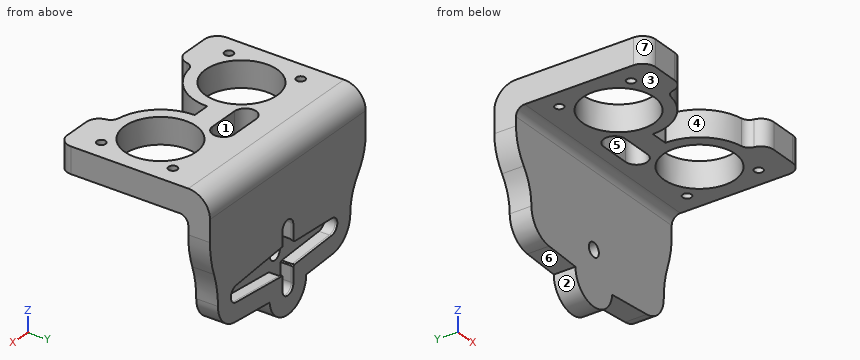
from build123d import *

# Parameters (mm, degrees)
EXTRUDE_THIN1_DEPTH = 5
BOSS_EXTRUDE1_DEPTH = 2
SKETCH3_R           = 1.6
CUT_EXTRUDE1_DEPTH  = 26.797771221
BOSS_EXTRUDE2_DEPTH = 5
SKETCH8_W           = 50
SKETCH8_H           = 6
BOSS_EXTRUDE6_DEPTH = 30
SKETCH10_R          = 8.25
SKETCH10_R_2        = 1
CUT_EXTRUDE2_DEPTH  = 55.037232534
FILLET2_R           = 5
FILLET4_R           = 3
EXTRUDE_THIN2_START = 4.5
EXTRUDE_THIN2_DEPTH = 0.5
FILLET5_R           = 2


# Read off the part's stored shape, not the designer's step: Extrude-Thin1, Boss-Extrude1, Extrude-Thin2
with BuildPart() as part:
    # Extrude-Thin1 outline → Extrude-Thin1 (new body)
    with BuildSketch(Plane(origin=(0, 0, 0), x_dir=(1, 0, 0), z_dir=(0, 1, 0))):
        with BuildLine():
            ThreePointArc((5.878005996, 6.958965141), (-0.252578975, 12.344591068), (-5.899998443, 6.454286146))
            Line((-5.899998443, 6.454286146), (-14.377365901, 5.991062641))
            ThreePointArc((-14.377365901, 5.991062641), (-20.05, 0), (-14.377365901, -5.991062641))
            Line((-14.377365901, -5.991062641), (-5.899998443, -6.454286146))
            ThreePointArc((-5.899998443, -6.454286146), (-0.252578975, -12.344591068), (5.878005996, -6.958965141))
            Line((5.878005996, -6.958965141), (16.97887538, -5.97664545))
            ThreePointArc((16.97887538, -5.97664545), (22.45, 0), (16.97887538, 5.97664545))
            Line((16.97887538, 5.97664545), (5.878005996, 6.958965141))
        make_face()
        with BuildLine():
            Line((-1.9, 2.87967012), (-1.9, 6.45))
            ThreePointArc((-1.9, 6.45), (0, 8.35), (1.9, 6.45))
            Line((1.9, 6.45), (1.9, 3.295349698))
            Line((1.9, 3.295349698), (16.626291793, 1.99221515))
            ThreePointArc((16.626291793, 1.99221515), (18.45, 0), (16.626291793, -1.99221515))
            Line((16.626291793, -1.99221515), (1.9, -3.295349698))
            Line((1.9, -3.295349698), (1.9, -6.45))
            ThreePointArc((1.9, -6.45), (0, -8.35), (-1.9, -6.45))
            Line((-1.9, -6.45), (-1.9, -2.87967012))
            ThreePointArc((-1.9, -2.87967012), (-2.057742861, -2.769150468), (-2.209072203, -2.65))
            Line((-2.209072203, -2.65), (-14.159121967, -1.99702088))
            ThreePointArc((-14.159121967, -1.99702088), (-16.05, 0), (-14.159121967, 1.99702088))
            Line((-14.159121967, 1.99702088), (-2.209072203, 2.65))
            ThreePointArc((-2.209072203, 2.65), (-2.057742861, 2.769150468), (-1.9, 2.87967012))
        make_face(mode=Mode.SUBTRACT)
    extrude(amount=EXTRUDE_THIN1_DEPTH)

    # Boss-Extrude1 outline → Boss-Extrude1 (add)
    with BuildSketch(Plane(origin=(0, 0, 0), x_dir=(1, 0, 0), z_dir=(0, 1, 0))):
        with BuildLine():
            ThreePointArc((1.9, 6.45), (0, 8.35), (-1.9, 6.45))
            Line((-1.9, 6.45), (-1.9, 2.87967012))
            ThreePointArc((-1.9, 2.87967012), (-2.057742861, 2.769150468), (-2.209072203, 2.65))
            Line((-2.209072203, 2.65), (-14.159121967, 1.99702088))
            ThreePointArc((-14.159121967, 1.99702088), (-16.05, 0), (-14.159121967, -1.99702088))
            Line((-14.159121967, -1.99702088), (-2.209072203, -2.65))
            ThreePointArc((-2.209072203, -2.65), (-2.057742861, -2.769150468), (-1.9, -2.87967012))
            Line((-1.9, -2.87967012), (-1.9, -6.45))
            ThreePointArc((-1.9, -6.45), (0, -8.35), (1.9, -6.45))
            Line((1.9, -6.45), (1.9, -3.295349698))
            Line((1.9, -3.295349698), (16.626291793, -1.99221515))
            ThreePointArc((16.626291793, -1.99221515), (18.45, 0), (16.626291793, 1.99221515))
            Line((16.626291793, 1.99221515), (1.9, 3.295349698))
            Line((1.9, 3.295349698), (1.9, 6.45))
        make_face()
    extrude(amount=BOSS_EXTRUDE1_DEPTH)

    # Sketch3 → Cut-Extrude1 (cut, through all)
    with BuildSketch(Plane(origin=(0, 2, 0), x_dir=(1, 0, 0), z_dir=(0, 1, 0))):
        with Locations(Location((0, 0, 0), (0, 0, 270))):
            Circle(SKETCH3_R)
    extrude(amount=-CUT_EXTRUDE1_DEPTH, mode=Mode.SUBTRACT)

    # Sketch4 → Boss-Extrude2 (add)
    # profile 1 of 2: a face of its own
    with BuildSketch(Plane.XZ):
        with BuildLine():
            Line((25, 25), (-25, 25))
            Line((-25, 25), (-25, 15))
            ThreePointArc((-25, 15), (-24.365263739, 11.051087966), (-22.525, 7.5))
            ThreePointArc((-22.525, 7.5), (-20.684736261, 3.948912034), (-20.05, 0))
            ThreePointArc((-20.05, 0), (-18.406844925, 4.125276027), (-14.377365901, 5.991062641))
            Line((-14.377365901, 5.991062641), (-5.899998443, 6.454286146))
            ThreePointArc((-5.899998443, 6.454286146), (-0.252578976, 12.344591068), (5.878005996, 6.958965141))
            Line((5.878005996, 6.958965141), (16.97887538, 5.97664545))
            ThreePointArc((16.97887538, 5.97664545), (20.875678043, 4.051342229), (22.45, 0))
            ThreePointArc((22.45, 0), (22.77102028, 3.803801552), (23.725, 7.5))
            ThreePointArc((23.725, 7.5), (24.67897972, 11.196198448), (25, 15))
            Line((25, 15), (25, 25))
        make_face()
    # profile 2 of 2: a face of its own
    with BuildSketch(Plane.XZ):
        with BuildLine():
            Line((-14.377365901, -5.991062641), (-5.899998443, -6.454286146))
            ThreePointArc((-5.899998443, -6.454286146), (-0.252578976, -12.344591068), (5.878005996, -6.958965141))
            Line((5.878005996, -6.958965141), (16.97887538, -5.97664545))
            ThreePointArc((16.97887538, -5.97664545), (22.45, 0), (16.97887538, 5.97664545))
            Line((16.97887538, 5.97664545), (5.878005996, 6.958965141))
            ThreePointArc((5.878005996, 6.958965141), (-0.252578976, 12.344591068), (-5.899998443, 6.454286146))
            Line((-5.899998443, 6.454286146), (-14.377365901, 5.991062641))
            ThreePointArc((-14.377365901, 5.991062641), (-20.05, 0), (-14.377365901, -5.991062641))
        make_face()
        with BuildLine():
            ThreePointArc((16.626291793, -1.99221515), (18.45, 0), (16.626291793, 1.99221515))
            Line((16.626291793, 1.99221515), (1.9, 3.295349698))
            Line((1.9, 3.295349698), (1.9, 6.45))
            ThreePointArc((1.9, 6.45), (0, 8.35), (-1.9, 6.45))
            Line((-1.9, 6.45), (-1.9, 2.87967012))
            ThreePointArc((-1.9, 2.87967012), (-2.057742862, 2.769150468), (-2.209072203, 2.65))
            Line((-2.209072203, 2.65), (-14.159121967, 1.99702088))
            ThreePointArc((-14.159121967, 1.99702088), (-16.05, 0), (-14.159121967, -1.99702088))
            Line((-14.159121967, -1.99702088), (-2.209072203, -2.65))
            ThreePointArc((-2.209072203, -2.65), (-2.057742862, -2.769150468), (-1.9, -2.87967012))
            Line((-1.9, -2.87967012), (-1.9, -6.45))
            ThreePointArc((-1.9, -6.45), (0, -8.35), (1.9, -6.45))
            Line((1.9, -6.45), (1.9, -3.295349698))
            Line((1.9, -3.295349698), (16.626291793, -1.99221515))
        make_face(mode=Mode.SUBTRACT)
    extrude(amount=-BOSS_EXTRUDE2_DEPTH)

    # Sketch8 → Boss-Extrude6 (add)
    with BuildSketch(Plane.XZ):
        with Locations((0, 22)):
            Rectangle(SKETCH8_W, SKETCH8_H)
    extrude(amount=BOSS_EXTRUDE6_DEPTH)

    # Sketch10 → Cut-Extrude2 (cut, through all)
    with BuildSketch(Plane.XY.offset(25)):
        with Locations((-13, -15)):
            Circle(SKETCH10_R)
        with Locations((13, -15)):
            Circle(SKETCH10_R)
        with Locations((20.5, -6.75)):
            Circle(SKETCH10_R_2)
        with Locations((20.5, -23.25)):
            Circle(SKETCH10_R_2)
        with Locations((-20.5, -23.25)):
            Circle(SKETCH10_R_2)
        with Locations((-20.5, -6.75)):
            Circle(SKETCH10_R_2)
        with BuildLine():
            Line((3.5, -9.8), (-3.5, -9.8))
            ThreePointArc((-3.5, -9.8), (-6, -7.3), (-3.5, -4.8))
            Line((-3.5, -4.8), (3.5, -4.8))
            ThreePointArc((3.5, -4.8), (6, -7.3), (3.5, -9.8))
        make_face()
        with BuildLine():
            Line((-2, -15), (2, -15))
            ThreePointArc((2, -15), (4.644900222, -22.154879991), (11.307692308, -25.869042951))
            ThreePointArc((11.307692308, -25.869042951), (12.519109051, -26.544345307), (13, -27.845232579))
            Line((13, -27.845232579), (13, -30))
            Line((13, -30), (-13, -30))
            Line((-13, -30), (-13, -27.845232579))
            ThreePointArc((-13, -27.845232579), (-12.519109051, -26.544345307), (-11.307692308, -25.869042951))
            ThreePointArc((-11.307692308, -25.869042951), (-4.644900222, -22.154879991), (-2, -15))
        make_face()
    extrude(amount=-CUT_EXTRUDE2_DEPTH, mode=Mode.SUBTRACT)

    # Fillet2
    fillet2_edges = [part.edges().sort_by_distance(p)[0] for p in [
        (0, 5, 25),
    ]]
    fillet(fillet2_edges, radius=FILLET2_R)

    # Fillet4
    fillet4_edges = [part.edges().sort_by_distance(p)[0] for p in [
        (25, -30, 22),
        (-25, -30, 22),
        (13, -30, 22),
        (-13, -30, 22),
    ]]
    fillet(fillet4_edges, radius=FILLET4_R)

    # Extrude-Thin2 outline → Extrude-Thin2 (add)
    with BuildSketch(Plane(origin=(0, 0, 0), x_dir=(1, 0, 0), z_dir=(0, 1, 0)).offset(EXTRUDE_THIN2_START)):
        with BuildLine():
            ThreePointArc((1.9, 6.45), (0, 8.35), (-1.9, 6.45))
            Line((-1.9, 6.45), (-1.9, 2.87967012))
            ThreePointArc((-1.9, 2.87967012), (-2.057742861, 2.769150468), (-2.209072203, 2.65))
            Line((-2.209072203, 2.65), (-14.159121967, 1.99702088))
            ThreePointArc((-14.159121967, 1.99702088), (-16.05, 0), (-14.159121967, -1.99702088))
            Line((-14.159121967, -1.99702088), (-2.209072203, -2.65))
            ThreePointArc((-2.209072203, -2.65), (-2.057742861, -2.769150468), (-1.9, -2.87967012))
            Line((-1.9, -2.87967012), (-1.9, -6.45))
            ThreePointArc((-1.9, -6.45), (0, -8.35), (1.9, -6.45))
            Line((1.9, -6.45), (1.9, -3.295349698))
            Line((1.9, -3.295349698), (16.626291793, -1.99221515))
            ThreePointArc((16.626291793, -1.99221515), (18.45, 0), (16.626291793, 1.99221515))
            Line((16.626291793, 1.99221515), (1.9, 3.295349698))
            Line((1.9, 3.295349698), (1.9, 6.45))
        make_face()
        with BuildLine():
            ThreePointArc((-1.75, -2.797766967), (-1.955868768, -2.657927268), (-2.150613493, -2.502970556))
            Line((-2.150613493, -2.502970556), (-14.15093782, -1.847244314))
            ThreePointArc((-14.15093782, -1.847244314), (-15.9, 0), (-14.15093782, 1.847244314))
            Line((-14.15093782, 1.847244314), (-2.150613493, 2.502970556))
            ThreePointArc((-2.150613493, 2.502970556), (-1.955868768, 2.657927268), (-1.75, 2.797766967))
            Line((-1.75, 2.797766967), (-1.75, 6.45))
            ThreePointArc((-1.75, 6.45), (0, 8.2), (1.75, 6.45))
            Line((1.75, 6.45), (1.75, 3.158037104))
            Line((1.75, 3.158037104), (16.613069909, 1.842799014))
            ThreePointArc((16.613069909, 1.842799014), (18.3, 0), (16.613069909, -1.842799014))
            Line((16.613069909, -1.842799014), (1.75, -3.158037104))
            Line((1.75, -3.158037104), (1.75, -6.45))
            ThreePointArc((1.75, -6.45), (0, -8.2), (-1.75, -6.45))
            Line((-1.75, -6.45), (-1.75, -2.797766967))
        make_face(mode=Mode.SUBTRACT)
    extrude(amount=EXTRUDE_THIN2_DEPTH)

    # Fillet5
    fillet5_edges = [part.edges().sort_by_distance(p)[0] for p in [
        (0, 0, 19),
    ]]
    fillet(fillet5_edges, radius=FILLET5_R)


solid = part.part
CAD build for the part. Positions are in the model's coordinates, mm. Face numbers are marked on the shaded views. A direction names the side the tool comes from. Round coordinates to 2 decimals unless told otherwise and drop trailing zeros. Write each loop counter-clockwise with the first axis right and the second up, starting at its lowest first coordinate (ties: lowest second). Pieces come first, ordered by that corner, then holes. Notation, with made-up numbers: M -19,-2.5 L -11,-2.5 A19 ccw -11,23.5 Z; hole C -17,83 d4. An arc over 180 degrees is marked long. Put each result on its own line as item: value. Start each with the question number.
1) Pin check, flat tips, straight feed: pin 1 Ø0.6 at (y, z) = (5, -4) entering from +X; pin 2 Ø0.6 at (y, z) = (5, 4.5) entering from +X; pin 3 Ø0.8 at (y, z) = (3, -5.5) entering from +X. Stop position of each tip, or through.
2) Saw through at A-A, the plane x = 0. Write the cut outline in (y, z).
3) Saw through at C-C, the plane x = 10. Write the cut outline in (y, z), and give its area (3 significant figures).
4) Saw through at B-B, the plane y = -21. Write the cut outline in (x, z).
5) 3-axis set-ups, long thin cutter, end or side, ignore diameter. For the marked faces 1, 2, 3 and 4: which of +Z, -Z, +X, -X, +Y, -Y reach the whole face in a straight line?
6) Pull direction Y, two halves, no side cores. Call the marked faces 5, 6 and 7: pulls with the +Y half, pulls with the -Y half, needs draft (parallel to the pull), parting line crosses it, or undercut.
7) Drill centre lines: probe 1 along X at (y, z) = (-6, 22); probe 2 along X at (y, z) = (-22.5, 20.5); probe 3 along Z at (x, y) = (-11, -25). Where is each one in solid material? Low to high. Write a range as [from, to].
8) Saw through at D-D, the plane z = -1. Write the cut outline in (x, y), and give its area (3 significant figures).
Resolved:
1. pin 1: x = 21.17
1. pin 2: x = 22.96
1. pin 3: x = 19.61
2. outline: M -15,19 L -9.8,19 L -9.8,25 L -15,25 Z; M -4.8,19 L -2,19 A2 cw 0,17 L 0,1.6 L 2,1.6 L 2,8.35 L 4.5,8.35 L 4.5,8.2 L 5,8.2 L 5,20 A5 ccw 0,25 L -4.8,25 Z; M 0,-12.35 L 5,-12.35 L 5,-8.2 L 4.5,-8.2 L 4.5,-8.35 L 2,-8.35 L 2,-1.6 L 0,-1.6 Z
3. outline: M -25.58,19 L -22.69,19 L -22.69,25 L -25.58,25 Z; M -7.31,19 L -2,19 A2 cw 0,17 L 0,-6.59 L 5,-6.59 L 5,-2.43 L 4.5,-2.43 L 4.5,-2.58 L 2,-2.58 L 2,2.58 L 4.5,2.58 L 4.5,2.43 L 5,2.43 L 5,20 A5 ccw 0,25 L -7.31,25 Z
3. area: 199 mm²
4. outline: M -25,19 L -18.66,19 L -18.66,25 L -25,25 Z; M -7.34,19 L -3.78,19 L -3.78,25 L -7.34,25 Z; M 3.78,19 L 7.34,19 L 7.34,25 L 3.78,25 Z; M 18.66,19 L 25,19 L 25,25 L 18.66,25 Z
5. face 1: +Z, -Z
5. face 2: -Z, +Y, -Y
5. face 3: -Z, +X, -X, -Y
5. face 4: +Z, -Z, -Y
6. face 5: undercut
6. face 6: needs draft
6. face 7: pulls with the -Y half
7. probe 1: [-25, -21.16], [-19.84, -5.64], [5.64, 19.84], [21.16, 25]
7. probe 2: [-25, -21.16], [-19.84, -16.44], [-9.56, -4.95], [4.95, 9.56], [16.44, 19.84], [21.16, 25]
7. probe 3: [19, 25]
8. outline: M -19.97,0 L -1.25,0 L -1.25,2 L -15.78,2 L -15.78,4.5 L -15.61,4.5 L -15.61,5 L -19.97,5 Z; M 1.25,0 L 22.37,0 L 22.37,5 L 18.01,5 L 18.01,4.5 L 18.18,4.5 L 18.18,2 L 1.25,2 Z
8. area: 105 mm²
